from build123d import *

# Parameters (mm, degrees)
BOSS_EXTRUDE1_DEPTH = 30
FILLET1_R           = 10
SKETCH2_R           = 10
CUT_EXTRUDE1_DEPTH  = 639.630555495


with BuildPart() as part:
    # Sketch1 → Boss-Extrude1 (new body)
    with BuildSketch(Plane(origin=(0, 0, 0), x_dir=(1, 0, 0), z_dir=(0, 1, 0))):
        Polygon((-637.611940299, 61.791044776), (-57.611940299, 61.791044776), (-57.611940299, 51.791044776), (2.388059701, 51.791044776), (2.388059701, 41.791044776), (-17.611940299, 41.791044776), (-637.611940299, 41.791044776), align=None)
    extrude(amount=BOSS_EXTRUDE1_DEPTH)

    # Fillet1
    fillet1_edges = [part.edges().sort_by_distance(p)[0] for p in [
        (2.388059701, 30, -46.791044776),
        (-57.611940299, 30, -56.791044776),
        (-57.611940299, 0, -56.791044776),
        (2.388059701, 0, -46.791044776),
    ]]
    fillet(fillet1_edges, radius=FILLET1_R)

    # Sketch2 → Cut-Extrude1 (cut, through all)
    with BuildSketch(Plane.XY.offset(-41.791044776)):
        with Locations((-21.046360359, 15)):
            Circle(SKETCH2_R)
        with Locations((-111.046360359, 15)):
            Circle(SKETCH2_R)
    extrude(amount=-CUT_EXTRUDE1_DEPTH, mode=Mode.SUBTRACT)


solid = part.part
The listing builds one solid part. Answer for the finished solid, in the listing's coordinates (mm). A direction names the side the tool comes from. Coordinates: 2 decimals unless noted, no trailing zeros. Order: outer loops, then holes, each group sorted by start corner. A loop starts at its lowest first (then second) coordinate and runs counter-clockwise, first axis right, second up.
Q1. A cutting plane is placed at A-A, the plane y = 15. Write down the section's boundary in (x, z).
Q2. For a pull along Y with two mould halves and no side action, classify faces 1 (the face through (-28.417, 21.758, -46.721)), 2 (the face through (-318, 0, -52)), 3 (the face through (-60.46, 26.99, -56.72)) as pulls with the +Y half, pulls with the -Y half, needs draft (parallel to the pull), parting line crosses it, or undercut.
Q3. Which of the six approach directions +Z, -Z, +X, -X, +Y, -Y give full straight-line access (tool end or side, diameter ignored) to faces 4 (the face through (-60.46, 3.01, -56.72)), 5 (the face through (2.388, 15, -47)), 6 (the face through (-57.612, 15, -57))?
Q4. Given P1, Ø12, axis at y = 3.5, z = -49, coming from the +X side; P2, Ø5, axis at y = 25, z = -56, coming from the +X side; P3, Ø15, axis at x = -48.5, y = 17.5, coming from the -Z side; P4, Ø18, axis at x = -111.05, y = 15, coming from the +Z side, each flat-ended and moving along its own axis, determine where each tip first touches the part or whether it passes through.
Q5. Consider line 1 (X direction, y = 17.25, z = -42.75); line 2 (X direction, y = 21, z = -48); line 3 (Y direction, x = -109.5, z = -50.25). Determine where each line is inside the solid, lowest interval first.
Answers follow:
1. outline: (-637.61, -61.79) - (-121.05, -61.79) - (-121.05, -41.79) - (-637.61, -41.79) - close; (-101.05, -61.79) - (-57.61, -61.79) - (-57.61, -51.79) - (-31.05, -51.79) - (-31.05, -41.79) - (-101.05, -41.79) - close; (-11.05, -51.79) - (2.39, -51.79) - (2.39, -41.79) - (-11.05, -41.79) - close
2. face 1: undercut
2. face 2: pulls with the -Y half
2. face 3: pulls with the +Y half
3. face 4: -Z, +X, -Y
3. face 5: +Z, -Z, +X, +Y, -Y
3. face 6: -Z, +X, +Y, -Y
4. P1: stops at x = 2.38
4. P2: stops at x = -57.93
4. P3: stops at z = -51.79
4. P4: passes through
5. line 1: x = -637.61 to -120.79, -101.3 to -30.79, -11.3 to 2.39
5. line 2: x = -637.61 to -119.05, -103.05 to -29.05, -13.05 to 2.34
5. line 3: y = 0 to 5.12, 24.88 to 30
